Source: CAD feature listing. Evaluate the final solid. Frame: model axes, mm. A direction names the side the tool comes from. Coordinates: 2 decimals unless noted, no trailing zeros. Order: outer loops, then holes, each group sorted by start corner. A loop starts at its lowest first (then second) coordinate and runs counter-clockwise, first axis right, second up.
```python
from build123d import *

# Parameters (mm, degrees)
SKETCH1_W                                    = 127
SKETCH1_H                                    = 34.925
SKETCH1_R                                    = 6.35
BOSS_EXTRUDE1_DEPTH                          = 9.525
CBORE_FOR_10_SOCKET_HEAD_CAP_SCREW1_AT_COUNT = 2
CBORE_FOR_10_SOCKET_HEAD_CAP_SCREW1_AT_PITCH = 27.477896212
CBORE_FOR_10_SOCKET_HEAD_CAP_SCREW1_2_COUNT  = 2
CBORE_FOR_10_SOCKET_HEAD_CAP_SCREW1_2_PITCH  = 57.404
CBORE_FOR_10_SOCKET_HEAD_CAP_SCREW1_3_COUNT  = 2
CBORE_FOR_10_SOCKET_HEAD_CAP_SCREW1_3_PITCH  = 82.586748551


with BuildPart() as part:
    # Sketch1 → Boss-Extrude1 (new body)
    with BuildSketch(Plane.XY):
        with Locations((0, 14.2875)):
            Rectangle(SKETCH1_W, SKETCH1_H)
        with Locations(Location((0, 6.35, 0), (0, 0, 180))):
            Circle(SKETCH1_R, mode=Mode.SUBTRACT)
    extrude(amount=BOSS_EXTRUDE1_DEPTH)

    # Sketch7 → CBORE for #10 Socket Head Cap Screw1 (revolve, cut)
    with BuildSketch(Plane(origin=(28.702, 21.082, 0), x_dir=(0, 1, 0), z_dir=(1, 0, 0))):
        Polygon((0, 0), (0, 9.525), (2.5527, 9.525), (2.5527, 4.826), (4.7625, 4.826), (4.7625, 0.635), (5.3975, 0), align=None)
    cbore_for_10_socket_head_cap_screw1 = revolve(axis=Axis((28.702, 21.082, -6.35), (0, 0, 1)), mode=Mode.SUBTRACT)

    # CBORE for #10 Socket Head Cap Screw1 at: CBORE for #10 Socket Head Cap Screw1 ×2
    with Locations(*[Vector(0.878160388030778, -0.47836631663781837, 0) * (i * CBORE_FOR_10_SOCKET_HEAD_CAP_SCREW1_AT_PITCH) for i in range(1, CBORE_FOR_10_SOCKET_HEAD_CAP_SCREW1_AT_COUNT)]):
        add(cbore_for_10_socket_head_cap_screw1, mode=Mode.SUBTRACT)

    # CBORE for _10 Socket Head Cap Screw1 2: CBORE for #10 Socket Head Cap Screw1 ×2
    with Locations(*[(-i * CBORE_FOR_10_SOCKET_HEAD_CAP_SCREW1_2_PITCH, 0, 0) for i in range(1, CBORE_FOR_10_SOCKET_HEAD_CAP_SCREW1_2_COUNT)]):
        add(cbore_for_10_socket_head_cap_screw1, mode=Mode.SUBTRACT)

    # CBORE for _10 Socket Head Cap Screw1 3: CBORE for #10 Socket Head Cap Screw1 ×2
    with Locations(*[Vector(-0.9872528151354362, -0.1591599164587503, 0) * (i * CBORE_FOR_10_SOCKET_HEAD_CAP_SCREW1_3_PITCH) for i in range(1, CBORE_FOR_10_SOCKET_HEAD_CAP_SCREW1_3_COUNT)]):
        add(cbore_for_10_socket_head_cap_screw1, mode=Mode.SUBTRACT)


solid = part.part
```
1. Material intervals for line 1 along X through (y, z) = (21, 1); line 2 along X through (y, z) = (17, 3.25); line 3 along X through (y, z) = (5, 2.5), sorted ascending.
2. Section query B-B, the plane z = 8.25. Count the separate pieces of the cut face and the enclosed holes in it, plus the area to 3 significant figures.
3. Section query A-A, the plane x = 0. Output: boundary loops of the cut face in (y, z) (3 decimals), plus the area to 3 significant figures.
4. Contact query for flat-ended pins moving along their axis: P1, Ø5, axis at x = -53, y = 7, coming from the -Z side; P2, Ø5, axis at x = -26.5, y = 22.5, coming from the -Z side. Output: stop coordinate, or through.
5. Access query for faces 5 (the cylindrical face through (-28.911, 16.324, 2.701)), 6 (the flat face through (63.5, 14, 5)). Directions: +Z, -Z, +X, -X, +Y, -Y. A direction counts if a zero-diameter tool reaches every point of the face in a straight line with its end or side. Return the directions, or none.
6. Draft query along X for faces 1 (the flat face through (-63.5, 14, 5)), 2 (the cylindrical face through (26.98, 19.2, 7.14)), 3 (the flat face through (-1, 31.75, 5)), 4 (the cylindrical face through (1.38, 12.55, 4.7)). Return one class per face: +X half, -X half, draft (parallel to the pull), parting line (faces both ways), or undercut.
Answer key:
1. line 1: x = -63.5 to -33.46, -23.94 to 23.94, 33.46 to 63.5
1. line 2: x = -63.5 to -31.16, -26.25 to 26.25, 31.16 to 63.5
1. line 3: x = -63.5 to -56.58, -49.08 to -6.2, 6.2 to 49.08, 56.58 to 63.5
2. separate pieces: 1
2. enclosed holes: 5
2. area: 4,230 mm2
3. outline: (-3.175, 0) - (0, 0) - (0, 9.525) - (-3.175, 9.525) - close; (12.7, 0) - (31.75, 0) - (31.75, 9.525) - (12.7, 9.525) - close
3. area: 212 mm2
4. P1: stops at z = 4.83
4. P2: stops at z = 0.28
5. face 5: -Z
5. face 6: +Z, -Z, +X, +Y, -Y
6. face 1: -X half
6. face 2: undercut
6. face 3: draft
6. face 4: undercut
